Source: CAD feature listing. Evaluate the final solid. Frame: model axes, mm. A direction names the side the tool comes from. Round coordinates to 2 decimals unless told otherwise and drop trailing zeros. Loops run counter-clockwise (first coordinate to the right, second up) from the corner with the lowest first, then second, coordinate; pieces in that order, holes last. Notation, with made-up numbers: M 47,-23.75 L 78,-23.75 A9 ccw 78,-7.75 Z; hole C 52.25,48.25 d6. An arc over 180 degrees is marked long. Answer as CSV lines item,"result". Start each with the question number.
Autodesk Inventor part; units mm, degrees
ref_plane "YZ Plane" through (0, 0, 0) normal (1, 0, 0) x (0, 1, 0)
ref_plane "XZ Plane" through (0, 0, 0) normal (0, 1, 0) x (-1, 0, 0)
ref_plane "XY Plane" through (0, 0, 0) normal (0, 0, 1) x (1, 0, 0)
sketch "スケッチ1" plane through (0, 0, 0) normal (0, 0, 1) x (1, 0, 0)
  circle A0 centre (0, 0) radius 16.9
  line L0 (-3, 13.1) -> (3, 13.1)
  line L1 (3, 13.1) -> (3, 16.9)
  line L2 (3, 16.9) -> (-3, 16.9)
  line L3 (-3, 16.9) -> (-3, 13.1)
  line L4 (-12.6, 5) -> (-16.9, 5)
  line L5 (-16.9, 5) -> (-16.9, -5)
  line L6 (-16.9, -5) -> (-12.6, -5)
  line L7 (-12.6, -5) -> (-12.6, 5)
  line L8 (16.9, 0) -> (-16.9, 0) construction
  line L9 (0, 16.9) -> (0, -16.9) construction
  line L10 (-3, -13.1) -> (3, -13.1)
  line L11 (3, -13.1) -> (3, -16.9)
  line L12 (3, -16.9) -> (-3, -16.9)
  line L13 (-3, -16.9) -> (-3, -13.1)
  line L14 (12.6, 5) -> (16.9, 5)
  line L15 (16.9, 5) -> (16.9, -5)
  line L16 (16.9, -5) -> (12.6, -5)
  line L17 (12.6, -5) -> (12.6, 5)
  point P0 (-12.6, 0)
  point P1 (0, 13.1)
  point P2 (-3, 16.6316)
  point P3 (-16.1434, 5)
  point P4 (-16.1434, -5)
  point P5 (-3, -16.6316)
  point P6 (3, -16.6316)
  point P7 (16.1434, -5)
  point P8 (16.1434, 5)
  point P9 (3, 16.6316)
  dimension "d0" = 33.8
  dimension "d1" = 6
  dimension "d2" = 10
  dimension "d3" = 3.8
  dimension "d4" = 4.3
extrude "押し出し1" add sketch "スケッチ1" along normal blind 4.4 contours L14 L17 L16 A0 L11 L10 L13 L6 L7 L4 L3 L0 L1
sketch "スケッチ2" plane through (0, 0, 0) normal (0, 0, -1) x (-1, 0, 0)
  circle A0 centre (0, 0) radius 15
  line L0 (12.8814, 7.6856) -> (10.9, 5.7042)
  line L1 (10.9, 5.7042) -> (10.9, -5.7042)
  line L2 (10.9, -5.7042) -> (12.8814, -7.6856)
  line L3 (12.6, 5) -> (12.6, -5)
  line L4 (15, 0) -> (-15, 0) construction
  line L5 (-6.0361, 13.7319) -> (-3.7042, 11.4)
  line L6 (-3.7042, 11.4) -> (3.7042, 11.4)
  line L7 (3.7042, 11.4) -> (6.0361, 13.7319)
  line L8 (0, 15) -> (0, -15) construction
  line L9 (-3, 13.1) -> (3, 13.1)
  line L10 (-12.8814, 7.6856) -> (-10.9, 5.7042)
  line L11 (-10.9, 5.7042) -> (-10.9, -5.7042)
  line L12 (-10.9, -5.7042) -> (-12.8814, -7.6856)
  line L13 (-6.0361, -13.7319) -> (-3.7042, -11.4)
  line L14 (-3.7042, -11.4) -> (3.7042, -11.4)
  line L15 (3.7042, -11.4) -> (6.0361, -13.7319)
  point P0 (-12.8814, 7.6856)
  point P1 (-12.8814, -7.6856)
  point P2 (-6.0361, -13.7319)
  point P3 (6.0361, -13.7319)
  dimension "d7" = 30
  dimension "d8" = 1.7
  dimension "d9" = 135
  dimension "d10" = 1.7
  dimension "d11" = 1.7
  dimension "d12" = 1.7
  dimension "d13" = 135
extrude "押し出し2" add sketch "スケッチ2" along normal blind 1.1 contours L0 L1 L2 A0 L15 L14 L13 L12 L11 L10 L5 L6 L7
sketch "スケッチ3" plane through (0, 0, -1.1) normal (0, 0, -1) x (-1, 0, 0)
  circle A0 centre (0, 0) radius 5.1
  dimension "d16" = 10.2
extrude "押し出し3" add sketch "スケッチ3" along normal blind 3
sketch "スケッチ4" plane through (0, 0, -4.1) normal (0, 0, -1) x (-1, 0, 0)
  point P0 (0, 0)
  point P1 (0, 0)
hole "穴1" at (0, 0, -4.1) direction (0, 0, 1) diameter 7.5 end through all
fillet "フィレット1" radius 1.1 16 edges at (-11.8907, 6.6949, -1.1) (-9.9301, 11.2424, -1.1) (-4.8701, 12.566, -1.1) (0, 11.4, -1.1) (4.8701, 12.566, -1.1) (9.9301, 11.2424, -1.1) (11.8907, 6.6949, -1.1) (10.9, 0, -1.1) (11.8907, -6.6949, -1.1) (9.9301, -11.2424, -1.1) (4.8701, -12.566, -1.1) (0, -11.4, -1.1) (-4.8701, -12.566, -1.1) (-9.9301, -11.2424, -1.1) (-11.8907, -6.6949, -1.1) (-10.9, 0, -1.1)
chamfer "面取り1" distance 1.5 angle 10 1 edges at (5.1, 0, -4.1) measured on face at (-5.0835, -0.4104, -3.1)
sketch "スケッチ5" plane through (0, 0, -1.1) normal (0, 0, -1) x (-1, 0, 0)
  line L0 (-3.0782, -8.4572) -> (3.0782, 8.4572)
  line L1 (0, -23.2842) -> (0, 23.2842)
  point P0 (0, 0)
  point P1 (0, 0)
  dimension "d30" = 18
  dimension "d31" = 20
hole "穴2" at (-3.0782, 8.4572, -1.1) at (3.0782, -8.4572, -1.1) direction (0, 0, 1) diameter 2.3 end through all
fillet "フィレット2" radius 0.5 2 edges at (3.0782, -9.6072, -1.1) (-3.0782, 7.3072, -1.1)
properties part number "555_Cap" material "鉄、鋳鉄"
1) Access query for faces 1 (the cylindrical face through (-4.962, -12.19, -0.786)), 2 (the cylindrical face through (10.569, -0.086, -0.786)), 3 (the flat face through (-12.6, 0, 2)), 4 (the cylindrical face through (4.91, 12.16, -0.77)), 5 (the flat face through (0, 12, 0)). Directions: +Z, -Z, +X, -X, +Y, -Y. A direction counts if a zero-diameter tool reaches every point of the face in a straight line with its end or side. Return the directions, or none.
2) Contact query for flat-ended pins moving along their axis: pin 1 Ø3 at (y, z) = (14.5, 1.5) entering from +X; pin 2 Ø3 at (y, z) = (14.5, 3) entering from -X; pin 3 Ø3 at (x, z) = (15, 1.5) entering from -Y. Output: stop coordinate, or through.
3) Section D-D, the plane y = -15. Return loops of the section in (x, z), and give its area (3 significant figures).
4) Ray query, line 1 along Y through (x, z) = (0, 1.25); line 2 along X through (y, z) = (0, 1.75); line 3 along Z through (x, y) = (-7, 5.5). Return the intervals inside material, ascending.
5) Mould query, pull axis X, two halves, no side actions, for faces 6 (the flat face through (3, 15, 2)), 7 (the cylindrical face through (-10.586, -0.086, -0.769)), 8 (the flat face through (14, -5, 2)). Classes: pulls with the +X half, pulls with the -X half, needs draft (parallel to the pull), parting line crosses it, or undercut.
6) Section C-C, the plane z = 1.25. Return loops of the section in (x, y), and give its area (3 significant figures).
Findings below:
1,face 1,"-Z, -Y"
1,face 2,"-Z, +X"
1,face 3,"+Z, -Z, -X"
1,face 4,"-Z, +Y"
1,face 5,"-Z"
2,pin 1,"x = 10.8"
2,pin 2,"x = -10.8"
2,pin 3,"y = -10.17"
3,outline,"M -7.79,0 L -3,0 L -3,4.4 L -7.79,4.4 Z; M 3,0 L 7.79,0 L 7.79,4.4 L 3,4.4 Z"
3,area,"42.1 mm²"
4,line 1,"-13.1 to -3.75, 3.75 to 13.1"
4,line 2,"-12.6 to -3.75, 3.75 to 12.6"
4,line 3,"-1.1 to 4.4"
5,face 6,"undercut"
5,face 7,"pulls with the -X half"
5,face 8,"needs draft"
6,outline,"M -16.14,-5 A16.9 ccw -3,-16.63 L -3,-13.1 L 3,-13.1 L 3,-16.63 A16.9 ccw 16.14,-5 L 12.6,-5 L 12.6,5 L 16.14,5 A16.9 ccw 3,16.63 L 3,13.1 L -3,13.1 L -3,16.63 A16.9 ccw -16.14,5 L -12.6,5 L -12.6,-5 Z; hole C -3.08,8.46 d2.3; hole C 0,0 d7.5; hole C 3.08,-8.46 d2.3"
6,area,"719 mm²"
